Work out the finished part from the listing and answer in its coordinate system (mm). A direction names the side the tool comes from. Round coordinates to 2 decimals unless told otherwise and drop trailing zeros. Loops run counter-clockwise (first coordinate to the right, second up) from the corner with the lowest first, then second, coordinate; pieces in that order, holes last.
```python
from build123d import *

# Parameters (mm, degrees)
SKETCH3_R           = 9.725108951
BOSS_EXTRUDE1_DEPTH = 7.62


with BuildPart() as part:
    # Sketch3 → Boss-Extrude1 (new body)
    # profile 1 of 3: a face of its own
    with BuildSketch(Plane.XY):
        with BuildLine():
            ThreePointArc((-107.617835055, -8.650731277), (-89.609901884, 0), (-107.617835055, 8.650731277))
            Line((-107.617835055, 8.650731277), (-107.617835055, 6.35))
            Line((-107.617835055, 6.35), (-100.691706912, 6.35))
            Line((-100.691706912, 6.35), (-96.881706912, 0))
            Line((-96.881706912, 0), (-100.691706912, -6.35))
            Line((-100.691706912, -6.35), (-107.617835055, -6.35))
            Line((-107.617835055, -6.35), (-107.617835055, -8.650731277))
        make_face()
    # profile 2 of 3: a face of its own
    with BuildSketch(Plane.XY):
        with BuildLine():
            ThreePointArc((-90.842848974, 5.08), (-89.609901884, 0), (-90.842848974, -5.08))
            Line((-90.842848974, -5.08), (-8.292848974, -5.08))
            ThreePointArc((-8.292848974, -5.08), (-9.725108951, 0), (-8.292848974, 5.08))
            Line((-8.292848974, 5.08), (-90.842848974, 5.08))
        make_face()
    # profile 3 of 3: a face of its own
    with BuildSketch(Plane.XY):
        Circle(SKETCH3_R)
        Polygon((3.666174209, -6.35), (7.332348419, 0), (3.666174209, 6.35), (-3.666174209, 6.35), (-7.332348419, 0), (-3.666174209, -6.35), align=None, mode=Mode.SUBTRACT)
    extrude(amount=BOSS_EXTRUDE1_DEPTH)


solid = part.part
```
1. Find section B-B (z = 2). Write down the section's boundary in (x, y).
Answer key:
outline: (-107.62, -8.65) arc R11.08 ccw to (-90.84, -5.08) - (-8.29, -5.08) arc R9.73 ccw (long way) to (-8.29, 5.08) - (-90.84, 5.08) arc R11.08 ccw to (-107.62, 8.65) - (-107.62, 6.35) - (-100.69, 6.35) - (-96.88, 0) - (-100.69, -6.35) - (-107.62, -6.35) - close; hole (-7.33, 0) - (-3.67, -6.35) - (3.67, -6.35) - (7.33, 0) - (3.67, 6.35) - (-3.67, 6.35) - close
2. Find section D-D (x = -70.5). Write down the section's boundary in (y, z), then the cut area to 3 significant figures.
Answer key:
outline: (-5.08, 0) - (5.08, 0) - (5.08, 7.62) - (-5.08, 7.62) - close
area: 77.4 mm2
3. Determine the mould class of faces 1 (the face through (-5.474, 3.219, 3.757)), 2 (the face through (-104, -6.35, 4)), 3 (the face through (-98.8, 3.2, 3.8)) for opening direction X: +X half, -X half, draft (parallel to the pull), parting line (faces both ways), or undercut.
Answer key:
face 1: undercut
face 2: draft
face 3: -X half
4. Which of the six approach directions +Z, -Z, +X, -X, +Y, -Y give full straight-line access (tool end or side, diameter ignored) to faces 4 (the face through (-50, -5.08, 4)), 5 (the face through (-49, 5.08, 4)), 6 (the face through (0, -6.35, 4)), 7 (the face through (-104, 6.35, 4))?
Answer key:
face 4: +Z, -Z, -Y
face 5: +Z, -Z, +Y
face 6: +Z, -Z
face 7: +Z, -Z, -X
5. Find section C-C (y = -2.5). Write down the section's boundary in (x, z).
Answer key:
outline: (-98.38, 0) - (-5.89, 0) - (-5.89, 7.62) - (-98.38, 7.62) - close; (5.89, 0) - (9.4, 0) - (9.4, 7.62) - (5.89, 7.62) - close
6. Find section A-A (x = 0). Write down the section's boundary in (y, z).
Answer key:
outline: (-9.73, 0) - (-6.35, 0) - (-6.35, 7.62) - (-9.73, 7.62) - close; (6.35, 0) - (9.73, 0) - (9.73, 7.62) - (6.35, 7.62) - close
7. Consider probe 1 along Y at (x, z) = (0.5, 7.25); probe 2 along X at (y, z) = (-5.5, 1); probe 3 along Y at (x, z) = (-88.5, 1.5). Determine where each line is inside the solid, lowest interval first.
Answer key:
probe 1: y = -9.71 to -6.35, 6.35 to 9.71
probe 2: x = -100.18 to -91.07, -8.02 to -4.16, 4.16 to 8.02
probe 3: y = -5.08 to 5.08
8. Given pin 1 (1 mm diameter, centred on x = -13, z = 4.5, fed in from -Y); pin 2 (3.5 mm diameter, centred on x = 1.5, z = 5, fed in from -Y); pin 3 (2 mm diameter, centred on x = -51, z = 5.5, fed in from +Y), each flat-ended and moving along its own axis, determine where each tip first touches the part or whether it passes through.
Answer key:
pin 1: stops at y = -5.08
pin 2: stops at y = -9.73
pin 3: stops at y = 5.08
